Read the model definition and answer for the solid it produces. Units are mm, in the model's axes. Face numbers are marked on the shaded views. A direction names the side the tool comes from. Coordinates: 2 decimals unless noted, no trailing zeros. Order: outer loops, then holes, each group sorted by start corner. A loop starts at its lowest first (then second) coordinate and runs counter-clockwise, first axis right, second up. Notation, with made-up numbers: M -16,-36.5 L 32,-36.5 A25 cw 32,-11.5 Z; hole C -20.75,63.25 d8. An arc over 180 degrees is marked long. Use a Markdown table: item, result. Add a question column.
1) Find section A-A on x = 0. Write down the section's boundary in (y, z).
2) The mould has two halves that part along X. Classify the marked faces 1, 2 and 3: released by +X, released by -X, zero draft, split by the parting line, or undercut.
3) Find the intervals of material crossed by probe 1 along X at (y, z) = (0, 15.25); probe 2 along Y at (x, z) = (19, 3.75); probe 3 along Y at (x, z) = (15, 6.25), in increasing order. Write a range as [from, to].
4) Find section B-B on y = 0. Write down the section's boundary in (x, z).
5) Each of these flat-tipped pins is pushed along its axis until it touches: pin 1 Ø1 at (x, z) = (6, 9.5) entering from +Y; pin 2 Ø2 at (x, y) = (12, 3.5) entering from +Z; pin 3 Ø3 at (x, z) = (-4, 11) entering from +Y; pin 4 Ø4 at (x, z) = (19, 7) entering from +Y. Where does it stop, or does it pass through?
6) Find section C-C on z = 7.75. Write down the section's boundary in (x, y).
7) Find section D-D on y = 8. Write down the section's boundary in (x, z), plus the area to 3 significant figures.
8) For the marked faces 4, 5 and 6, determine the directions among +Z, -Z, +X, -X, +Y, -Y from which every point of the face is accessible in a straight line to the end or side of a thin tool.
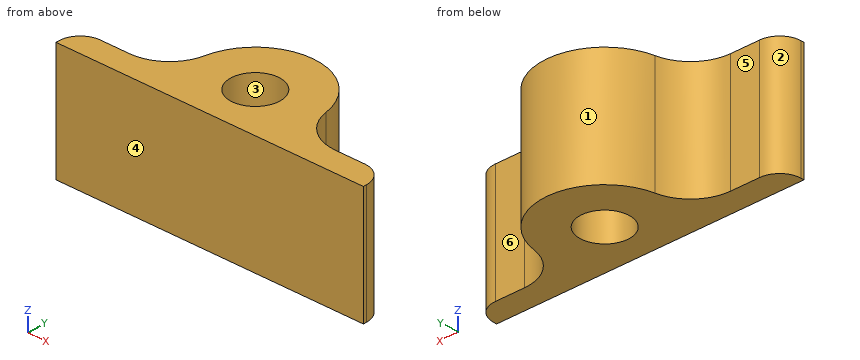
Autodesk Fusion 360 part; units mm, degrees
sketch "Sketch1" plane through (0, 0, 0) normal (0, 0, 1) x (1, 0, 0)
  circle A0 centre (0, 0) radius 4
  circle A1 centre (0, 0) radius 10
  line L0 (-25, -8) -> (25, -8)
  line L1 (25, -8) -> (25, -4)
  line L2 (25, -4) -> (-25, -4)
  line L3 (-25, -4) -> (-25, -8)
  line L4 (-25, -8) -> (25, -4) construction
  line L5 (25, -8) -> (-25, -4) construction
  circle A2 centre (-16.7332, 3) radius 7
  circle A3 centre (16.7332, 3) radius 7
  dimension "d1" = 8
  dimension "d2" = 20
  dimension "d3" = 50
  dimension "d4" = 4
  dimension "d5" = 14
  dimension "d6" = 14
extrude "Extrude1" add sketch "Sketch1" along normal blind 19 contours A1 L2 | A1 L0 L2 | A1 L0 L1 L2 | A1 L2 A3 | A1 L2 A2 | A1 L0 L2 L3
fillet "Fillet1" radius 3.5 2 edges at (25, -4, 9.5) (-25, -4, 9.5)
Check result:
| question | item | result |
|---|---|---|
| 1 | outline | M -8,0 L -4,0 L -4,19 L -8,19 Z; M 4,0 L 10,0 L 10,19 L 4,19 Z |
| 2 | face 1 | split by the parting line |
| 2 | face 2 | released by -X |
| 2 | face 3 | undercut |
| 3 | probe 1 | x = [-10.41, -4], [4, 10.41] |
| 3 | probe 2 | y = [-8, -4] |
| 3 | probe 3 | y = [-8, -3.78] |
| 4 | outline | M -10.41,0 L -4,0 L -4,19 L -10.41,19 Z; M 4,0 L 10.41,0 L 10.41,19 L 4,19 Z |
| 5 | pin 1 | stops at y = 8.35 |
| 5 | pin 2 | passes through |
| 5 | pin 3 | stops at y = 9.68 |
| 5 | pin 4 | stops at y = -4 |
| 6 | outline | M -25,-8 L 25,-8 L 25,-7.5 A3.5 ccw 21.5,-4 L 16.73,-4 A7 cw 9.84,1.76 A10 ccw -9.84,1.76 A7 cw -16.73,-4 L -21.5,-4 A3.5 ccw -25,-7.5 Z; hole C 0,0 d8 |
| 7 | outline | M -6,0 L 6,0 L 6,19 L -6,19 Z |
| 7 | area | 228 mm2 |
| 8 | face 4 | +Z, -Z, +X, -X, -Y |
| 8 | face 5 | +Z, -Z, -X, +Y |
| 8 | face 6 | +Z, -Z, +X, +Y |
